Input: part model. Units: mm. Frame: model coordinates. A direction names the side the tool comes from. Give positions to 0.01 mm unless a question says otherwise; leave off trailing zeros. Answer as a JSON object with one key per item and string values.
```python
from build123d import *

# Parameters (mm, degrees)
EXTRUDE1_DEPTH = 203.2


with BuildPart() as part:
    # Sketch1 → Extrude1 (new body)
    with BuildSketch(Plane.XY):
        with BuildLine():
            Line((-3.88464389, 5.447103113), (-7.193320288, 8.75577951))
            ThreePointArc((-7.193320288, 8.75577951), (-7.413561403, 9.863006367), (-6.474899798, 10.4902))
            Line((-6.474899798, 10.4902), (-4.3561, 10.4902))
            ThreePointArc((-4.3561, 10.4902), (-3.2512, 11.5951), (-4.3561, 12.7))
            Line((-4.3561, 12.7), (-10.5918, 12.7))
            ThreePointArc((-10.5918, 12.7), (-12.082522516, 12.082522516), (-12.7, 10.5918))
            Line((-12.7, 10.5918), (-12.7, 4.3561))
            ThreePointArc((-12.7, 4.3561), (-11.5951, 3.2512), (-10.4902, 4.3561))
            Line((-10.4902, 4.3561), (-10.4902, 6.474899798))
            ThreePointArc((-10.4902, 6.474899798), (-9.863006367, 7.413561403), (-8.75577951, 7.193320288))
            Line((-8.75577951, 7.193320288), (-5.447103113, 3.88464389))
            ThreePointArc((-5.447103113, 3.88464389), (-4.758849627, 2.854599758), (-4.517167143, 1.63957986))
            Line((-4.517167143, 1.63957986), (-4.517167143, -1.63957986))
            ThreePointArc((-4.517167143, -1.63957986), (-4.758849627, -2.854599758), (-5.447103113, -3.88464389))
            Line((-5.447103113, -3.88464389), (-8.75577951, -7.193320288))
            ThreePointArc((-8.75577951, -7.193320288), (-9.863006367, -7.413561403), (-10.4902, -6.474899798))
            Line((-10.4902, -6.474899798), (-10.4902, -4.3561))
            ThreePointArc((-10.4902, -4.3561), (-11.5951, -3.2512), (-12.7, -4.3561))
            Line((-12.7, -4.3561), (-12.7, -10.5918))
            ThreePointArc((-12.7, -10.5918), (-12.082522516, -12.082522516), (-10.5918, -12.7))
            Line((-10.5918, -12.7), (-4.3561, -12.7))
            ThreePointArc((-4.3561, -12.7), (-3.2512, -11.5951), (-4.3561, -10.4902))
            Line((-4.3561, -10.4902), (-6.474899798, -10.4902))
            ThreePointArc((-6.474899798, -10.4902), (-7.413561403, -9.863006367), (-7.193320288, -8.75577951))
            Line((-7.193320288, -8.75577951), (-3.88464389, -5.447103113))
            ThreePointArc((-3.88464389, -5.447103113), (-2.854599758, -4.758849627), (-1.63957986, -4.517167143))
            Line((-1.63957986, -4.517167143), (1.63957986, -4.517167143))
            ThreePointArc((1.63957986, -4.517167143), (2.854599758, -4.758849627), (3.88464389, -5.447103113))
            Line((3.88464389, -5.447103113), (7.193320288, -8.75577951))
            ThreePointArc((7.193320288, -8.75577951), (7.413561403, -9.863006367), (6.474899798, -10.4902))
            Line((6.474899798, -10.4902), (4.3561, -10.4902))
            ThreePointArc((4.3561, -10.4902), (3.2512, -11.5951), (4.3561, -12.7))
            Line((4.3561, -12.7), (10.5918, -12.7))
            ThreePointArc((10.5918, -12.7), (12.082522516, -12.082522516), (12.7, -10.5918))
            Line((12.7, -10.5918), (12.7, -4.3561))
            ThreePointArc((12.7, -4.3561), (11.5951, -3.2512), (10.4902, -4.3561))
            Line((10.4902, -4.3561), (10.4902, -6.474899798))
            ThreePointArc((10.4902, -6.474899798), (9.863006367, -7.413561403), (8.75577951, -7.193320288))
            Line((8.75577951, -7.193320288), (5.447103113, -3.88464389))
            ThreePointArc((5.447103113, -3.88464389), (4.758849627, -2.854599758), (4.517167143, -1.63957986))
            Line((4.517167143, -1.63957986), (4.517167143, 1.63957986))
            ThreePointArc((4.517167143, 1.63957986), (4.758849627, 2.854599758), (5.447103113, 3.88464389))
            Line((5.447103113, 3.88464389), (8.75577951, 7.193320288))
            ThreePointArc((8.75577951, 7.193320288), (9.863006367, 7.413561403), (10.4902, 6.474899798))
            Line((10.4902, 6.474899798), (10.4902, 4.3561))
            ThreePointArc((10.4902, 4.3561), (11.5951, 3.2512), (12.7, 4.3561))
            Line((12.7, 4.3561), (12.7, 10.5918))
            ThreePointArc((12.7, 10.5918), (12.082522516, 12.082522516), (10.5918, 12.7))
            Line((10.5918, 12.7), (4.3561, 12.7))
            ThreePointArc((4.3561, 12.7), (3.2512, 11.5951), (4.3561, 10.4902))
            Line((4.3561, 10.4902), (6.474899798, 10.4902))
            ThreePointArc((6.474899798, 10.4902), (7.413561403, 9.863006367), (7.193320288, 8.75577951))
            Line((7.193320288, 8.75577951), (3.88464389, 5.447103113))
            ThreePointArc((3.88464389, 5.447103113), (2.854599758, 4.758849627), (1.63957986, 4.517167143))
            Line((1.63957986, 4.517167143), (-1.63957986, 4.517167143))
            ThreePointArc((-1.63957986, 4.517167143), (-2.854599758, 4.758849627), (-3.88464389, 5.447103113))
        make_face()
        with BuildLine():
            Line((-2.860474191, -1.969151357), (-2.231856263, -1.340533428))
            ThreePointArc((-2.231856263, -1.340533428), (-2.6035, 0), (-2.231856263, 1.340533428))
            Line((-2.231856263, 1.340533428), (-2.860474191, 1.969151357))
            ThreePointArc((-2.860474191, 1.969151357), (-2.918583239, 2.918583239), (-1.969151357, 2.860474191))
            Line((-1.969151357, 2.860474191), (-1.340533428, 2.231856263))
            ThreePointArc((-1.340533428, 2.231856263), (0, 2.6035), (1.340533428, 2.231856263))
            Line((1.340533428, 2.231856263), (1.969151357, 2.860474191))
            ThreePointArc((1.969151357, 2.860474191), (2.918583239, 2.918583239), (2.860474191, 1.969151357))
            Line((2.860474191, 1.969151357), (2.231856263, 1.340533428))
            ThreePointArc((2.231856263, 1.340533428), (2.6035, 0), (2.231856263, -1.340533428))
            Line((2.231856263, -1.340533428), (2.860474191, -1.969151357))
            ThreePointArc((2.860474191, -1.969151357), (2.918583239, -2.918583239), (1.969151357, -2.860474191))
            Line((1.969151357, -2.860474191), (1.340533428, -2.231856263))
            ThreePointArc((1.340533428, -2.231856263), (0, -2.6035), (-1.340533428, -2.231856263))
            Line((-1.340533428, -2.231856263), (-1.969151357, -2.860474191))
            ThreePointArc((-1.969151357, -2.860474191), (-2.918583239, -2.918583239), (-2.860474191, -1.969151357))
        make_face(mode=Mode.SUBTRACT)
    extrude(amount=-EXTRUDE1_DEPTH)


solid = part.part
```
Q1. Draft query along Y for faces 5 (the flat face through (12.7, -8, -100)), 6 (the flat face through (8, 12.7, -100)), 7 (the flat face through (-5.52, 7.08, -100.18)). Return one class per face: +Y half, -Y half, draft (parallel to the pull), parting line (faces both ways), or undercut.
Evaluation:
{"face 5": "draft", "face 6": "+Y half", "face 7": "undercut"}
Q2. Pin query (flat end, axial travel): pin 1 (1.6 mm diameter, centred on y = -0.5, z = -76, fed in from -X); pin 2 (2.5 mm diameter, centred on x = 0.5, z = -122.5, fed in from -Y); pin 3 (3.5 mm diameter, centred on x = 0, z = -125.5, fed in from +Y); pin 4 (2 mm diameter, centred on x = 2, y = 3.5, fed in from +Z). Return the tip coordinate at first contact, or that it passes through.
Evaluation:
{"pin 1": "stops at x = -4.52", "pin 2": "stops at y = -4.52", "pin 3": "stops at y = 4.52", "pin 4": "stops at z = 0"}
Q3. Access query for faces 1 (the flat face through (0, 4.517, -100)), 2 (the flat face through (4.517, 0, -100)), 3 (the flat face through (0, -4.517, -100)), 4 (the flat face through (7.08, 5.52, -100.18)). Directions: +Z, -Z, +X, -X, +Y, -Y. A direction counts if a zero-diameter tool reaches every point of the face in a straight line with its end or side. Return the directions, or none.
Evaluation:
{"face 1": "+Z, -Z, +Y", "face 2": "+Z, -Z, +X", "face 3": "+Z, -Z, -Y", "face 4": "+Z, -Z"}
Q4. Ray query, line 1 along Y through (x, z) = (-3.5, -15.5); line 2 along X through (y, z) = (9.75, -82); line 3 along X through (y, z) = (0, -157). Return the intervals inside material, ascending.
Evaluation:
{"line 1": "y = -12.29 to -10.9, -5.12 to 5.12, 10.9 to 12.29", "line 2": "x = -12.7 to -7.45, 7.45 to 12.7", "line 3": "x = -4.52 to -2.6, 2.6 to 4.52"}
